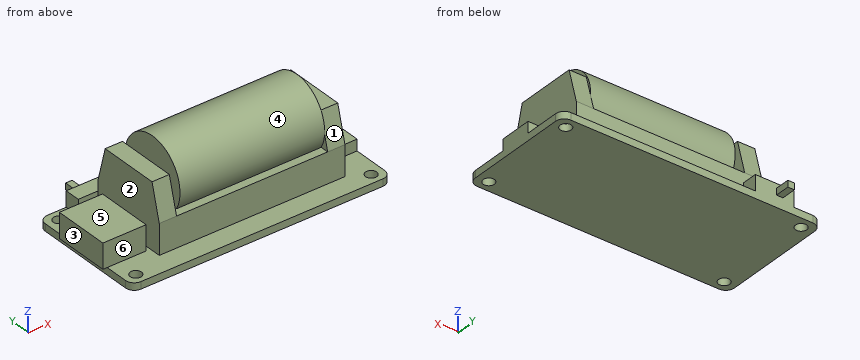
Autodesk Fusion 360 part; units mm, degrees
sketch "Sketch1" plane through (0, 0, 0) normal (0, 0, 1) x (1, 0, 0)
  line L0 (2, 0) -> (58, 0)
  line L1 (60, 2) -> (60, 26)
  line L2 (58, 28) -> (2, 28)
  line L3 (0, 26) -> (0, 2)
  arc A0 (2, 28) -> (0, 26) centre (2, 26) ccw
  arc A1 (60, 26) -> (58, 28) centre (58, 26) ccw
  arc A2 (58, 0) -> (60, 2) centre (58, 2) ccw
  arc A3 (0, 2) -> (2, 0) centre (2, 2) ccw
  point P0 (60, 0)
  point P1 (0, 28)
  dimension "d56" = 60
  dimension "d57" = 28
  dimension "d58" = 2
extrude "Extrude1" add sketch "Sketch1" along normal blind 1.65
sketch "Sketch2" plane through (0, 0, 1.65) normal (0, 0, 1) x (-1, 0, 0)
  arc A0 (0, -2) -> (-2, 0) centre (-2, -2) ccw
  line L0 (-2, 0) -> (-58, 0)
  arc A1 (-58, 0) -> (-60, -2) centre (-58, -2) ccw
  line L1 (-60, -2) -> (-60, -26)
  arc A2 (-60, -26) -> (-58, -28) centre (-58, -26) ccw
  line L2 (-58, -28) -> (-2, -28)
  arc A3 (-2, -28) -> (0, -26) centre (-2, -26) ccw
  line L3 (0, -26) -> (0, -2)
  line L4 (1, -20.5) -> (-9, -20.5)
  line L5 (-9, -20.5) -> (-9, -7.5)
  line L6 (-9, -7.5) -> (1, -7.5)
  line L7 (1, -7.5) -> (1, -20.5)
  line L8 (0, -14) -> (-60, -14) construction
  dimension "d61" = 10
  dimension "d62" = 13
  dimension "d63" = 1
extrude "Extrude2" add sketch "Sketch2" along normal blind 5.75 contours L3 L4 L6 L7 | L3 L4 L5 L6
sketch "Sketch3" plane through (0, 0, 1.65) normal (0, 0, 1) x (-1, 0, 0)
  line L0 (-9, -7.5) -> (0, -7.5)
  line L1 (0, -7.5) -> (0, -2)
  arc A0 (0, -2) -> (-2, 0) centre (-2, -2) ccw
  line L2 (-2, 0) -> (-58, 0)
  arc A1 (-58, 0) -> (-60, -2) centre (-58, -2) ccw
  line L3 (-60, -2) -> (-60, -26)
  arc A2 (-60, -26) -> (-58, -28) centre (-58, -26) ccw
  line L4 (-58, -28) -> (-2, -28)
  arc A3 (-2, -28) -> (0, -26) centre (-2, -26) ccw
  line L5 (0, -26) -> (0, -20.5)
  line L6 (0, -20.5) -> (-9, -20.5)
  line L7 (-9, -20.5) -> (-9, -7.5)
  line L8 (-9, -14) -> (-60, -14) construction
  line L9 (-10, -23.15) -> (-53, -23.15)
  line L10 (-53, -23.15) -> (-53, -4.85)
  line L11 (-53, -4.85) -> (-10, -4.85)
  line L12 (-10, -4.85) -> (-10, -23.15)
  dimension "d66" = 43
  dimension "d67" = 18.3
  dimension "d68" = 1
extrude "Extrude3" add sketch "Sketch3" along normal blind 15 contours L9 L10 L11 L12
sketch "Sketch4" plane through (53, 0, 0) normal (1, 0, 0) x (0, 1, 0)
  line L0 (4.85, 1.65) -> (23.15, 1.65)
  line L1 (23.15, 1.65) -> (23.15, 16.65)
  line L2 (23.15, 16.65) -> (4.85, 16.65)
  line L3 (4.85, 16.65) -> (4.85, 1.65)
  line L4 (4.85, 8.65) -> (7.2688, 17.65)
  line L5 (7.2688, 17.65) -> (20.7313, 17.65)
  line L6 (20.7313, 17.65) -> (23.15, 8.65)
  line L7 (4.85, 8.65) -> (23.15, 8.65) construction
  line L8 (7, 16.65) -> (21, 16.65) construction
  line L9 (14, 16.65) -> (14, 1.65) construction
  dimension "d71" = 14
  dimension "d72" = 7
  dimension "d73" = 1
extrude "Extrude4" cut sketch "Sketch4" against normal up to surface (43 mm away) contours L2 L3 L4 | L1 L2 L6
sketch "Sketch5" plane through (0, 4.85, 0) normal (0, -1, 0) x (1, 0, 0)
  line L0 (53, 8.65) -> (10, 8.65)
  line L1 (10, 8.65) -> (10, 1.65)
  line L2 (10, 1.65) -> (53, 1.65)
  line L3 (53, 1.65) -> (53, 8.65)
  line L4 (14, 16.65) -> (49, 16.65)
  line L5 (49, 16.65) -> (49, 8.65)
  line L6 (49, 8.65) -> (14, 8.65)
  line L7 (14, 8.65) -> (14, 16.65)
  line L8 (10, 8.65) -> (10, 16.65)
  line L9 (31.5, 1.65) -> (31.5, 16.653) construction
  line L10 (10, 16.65) -> (53, 16.65) construction
  dimension "d76" = 4
extrude "Extrude5" cut sketch "Sketch5" against normal through all contours L0 L4 L5 L6 L7
sketch "Sketch6" plane through (0, 0, 8.65) normal (0, 0, 1) x (-1, 0, 0)
  line L0 (-49, -23.15) -> (-14, -23.15)
  line L1 (-14, -23.15) -> (-14, -4.85)
  line L2 (-14, -4.85) -> (-49, -4.85)
  line L3 (-49, -4.85) -> (-49, -23.15)
  line L4 (-14, -14) -> (-49, -14) construction
  line L5 (-14, -21.15) -> (-49, -21.15)
  line L6 (-49, -21.15) -> (-49, -6.85)
  line L7 (-49, -6.85) -> (-14, -6.85)
  line L8 (-14, -6.85) -> (-14, -21.15)
  dimension "d78" = 2
extrude "Extrude6" cut sketch "Sketch6" against normal blind 6 contours L1 L3 L5 L6 L7 L8
sketch "Sketch7" plane through (49, 0, 0) normal (-1, 0, 0) x (0, -1, 0)
  line L0 (-4.85, 8.65) -> (-7, 16.65)
  line L1 (-7, 16.65) -> (-21, 16.65)
  line L2 (-21, 16.65) -> (-23.15, 8.65)
  line L3 (-23.15, 8.65) -> (-21.15, 8.65)
  line L4 (-21.15, 8.65) -> (-21.15, 2.65)
  line L5 (-21.15, 2.65) -> (-6.85, 2.65)
  line L6 (-6.85, 2.65) -> (-6.85, 8.65)
  line L7 (-6.85, 8.65) -> (-4.85, 8.65)
  line L8 (-14, 16.65) -> (-14, 2.65) construction
  circle A0 centre (-14, 12.65) radius 8.25
  dimension "d81" = 16.5
  dimension "d82" = 4
extrude "Extrude7" add sketch "Sketch7" along normal blind 33.5 contours L0 L1 L2 L3 L4 L6 L7 A0 | L0 L1 L2 A0
sketch "Sketch8" plane through (0, 0, 1.65) normal (0, 0, 1) x (-1, 0, 0)
  line L0 (-10, -4.85) -> (-10, -23.15)
  line L1 (-10, -23.15) -> (-53, -23.15)
  line L2 (-53, -23.15) -> (-53, -4.85)
  line L3 (-53, -4.85) -> (-10, -4.85)
  line L4 (-9, -7.5) -> (0, -7.5)
  line L5 (0, -7.5) -> (0, -2)
  arc A0 (0, -2) -> (-2, 0) centre (-2, -2) ccw
  line L6 (-2, 0) -> (-58, 0)
  arc A1 (-58, 0) -> (-60, -2) centre (-58, -2) ccw
  line L7 (-60, -2) -> (-60, -26)
  arc A2 (-60, -26) -> (-58, -28) centre (-58, -26) ccw
  line L8 (-58, -28) -> (-2, -28)
  arc A3 (-2, -28) -> (0, -26) centre (-2, -26) ccw
  line L9 (0, -26) -> (0, -20.5)
  line L10 (0, -20.5) -> (-9, -20.5)
  line L11 (-9, -20.5) -> (-9, -7.5)
  line L12 (-60, -14) -> (-9, -14) construction
  line L13 (-60, -17.75) -> (-54.4, -17.75)
  line L14 (-54.4, -17.75) -> (-54.4, -10.25)
  line L15 (-54.4, -10.25) -> (-60, -10.25)
  line L16 (-60, -10.25) -> (-60, -17.75)
  dimension "d85" = 5.6
  dimension "d86" = 7.5
extrude "Extrude8" add sketch "Sketch8" along normal blind 2.6 contours L7 L13 L14 L15 L16
sketch "Sketch9" plane through (0, 0, 0) normal (0, 0, -1) x (1, 0, 0)
  arc A0 (2, 0) -> (0, -2) centre (2, -2) ccw
  line L0 (0, -2) -> (0, -26)
  arc A1 (0, -26) -> (2, -28) centre (2, -26) ccw
  line L1 (2, -28) -> (58, -28)
  arc A2 (58, -28) -> (60, -26) centre (58, -26) ccw
  line L2 (60, -26) -> (60, -2)
  arc A3 (60, -2) -> (58, 0) centre (58, -2) ccw
  line L3 (58, 0) -> (2, 0)
  line L4 (0, -14) -> (60, -14) construction
  line L5 (30, 0) -> (30, -28) construction
  circle A4 centre (2.75, -2.5) radius 1.3
  circle A5 centre (57.25, -2.5) radius 1.3
  circle A6 centre (2.75, -25.5) radius 1.3
  circle A7 centre (57.25, -25.5) radius 1.3
  line L6 (2.75, -2.5) -> (57.25, -2.5) construction
  line L7 (57.25, -2.5) -> (57.25, -25.5) construction
  line L8 (57.25, -25.5) -> (2.75, -25.5) construction
  line L9 (2.75, -25.5) -> (2.75, -2.5) construction
  dimension "d89" = 23
  dimension "d90" = 54.5
  dimension "d91" = 2.6
extrude "Extrude9" cut sketch "Sketch9" against normal up to surface (1.65 mm away) contours A4 | A5 | A6 | A7
sketch "Sketch10" plane through (0, 0, 1.65) normal (0, 0, 1) x (-1, 0, 0)
  circle A0 centre (-57.25, -2.5) radius 1.3
  circle A1 centre (-57.25, -25.5) radius 1.3
  circle A2 centre (-2.75, -2.5) radius 1.3
  circle A3 centre (-2.75, -25.5) radius 1.3
  line L0 (-54.4, -17.75) -> (-60, -17.75)
  line L1 (-60, -17.75) -> (-60, -26)
  arc A4 (-60, -26) -> (-58, -28) centre (-58, -26) ccw
  line L2 (-58, -28) -> (-2, -28)
  arc A5 (-2, -28) -> (0, -26) centre (-2, -26) ccw
  line L3 (0, -26) -> (0, -20.5)
  line L4 (0, -20.5) -> (-9, -20.5)
  line L5 (-9, -20.5) -> (-9, -7.5)
  line L6 (-9, -7.5) -> (0, -7.5)
  line L7 (0, -7.5) -> (0, -2)
  arc A6 (0, -2) -> (-2, 0) centre (-2, -2) ccw
  line L8 (-2, 0) -> (-58, 0)
  arc A7 (-58, 0) -> (-60, -2) centre (-58, -2) ccw
  line L9 (-60, -2) -> (-60, -10.25)
  line L10 (-60, -10.25) -> (-54.4, -10.25)
  line L11 (-54.4, -10.25) -> (-54.4, -17.75)
  line L12 (-10, -4.85) -> (-10, -23.15)
  line L13 (-10, -23.15) -> (-53, -23.15)
  line L14 (-53, -23.15) -> (-53, -4.85)
  line L15 (-53, -4.85) -> (-10, -4.85)
  line L16 (-6.4, -28) -> (-15.3, -28)
  line L17 (-15.3, -28) -> (-15.3, -24.4)
  line L18 (-15.3, -24.4) -> (-6.4, -24.4)
  line L19 (-6.4, -24.4) -> (-6.4, -28)
  dimension "d1" = 8.9
  dimension "d2" = 3.6
  dimension "d3" = 15.3
extrude "Extrude10" add sketch "Sketch10" along normal blind 3.6 contours L2 L16 L17 L18 L19
sketch "Sketch11" plane through (0, 28, 0) normal (0, 1, 0) x (-1, 0, 0)
  line L0 (-58, 0) -> (-2, 0)
  line L1 (-2, 0) -> (-2, 1.65)
  line L2 (-2, 1.65) -> (-6.4, 1.65)
  line L3 (-6.4, 1.65) -> (-6.4, 5.25)
  line L4 (-6.4, 5.25) -> (-15.3, 5.25)
  line L5 (-15.3, 5.25) -> (-15.3, 1.65)
  line L6 (-15.3, 1.65) -> (-58, 1.65)
  line L7 (-58, 1.65) -> (-58, 0)
  line L8 (-15.3, 3.45) -> (-6.4, 3.45) construction
  line L9 (-8.9, 2.7) -> (-10.4, 2.7)
  line L10 (-10.4, 2.7) -> (-10.4, 4.2)
  line L11 (-10.4, 4.2) -> (-8.9, 4.2)
  line L12 (-8.9, 4.2) -> (-8.9, 2.7)
  line L13 (-8.9, 2.7) -> (-10.4, 4.2) construction
  line L14 (-10.4, 2.7) -> (-8.9, 4.2) construction
  point P0 (-9.65, 3.45)
  dimension "d6" = 1.5
  dimension "d7" = 1.5
  dimension "d8" = 2.5
extrude "Extrude11" add sketch "Sketch11" along normal blind 3.4 contours L9 L10 L11 L12
Check sheet for the modelled part. Datum: model origin and axes. Units: mm. Face numbers are marked on the shaded views. A direction names the side the tool comes from. Round coordinates to 2 decimals unless told otherwise and drop trailing zeros. Order: outer loops, then holes, each group sorted by start corner. A loop starts at its lowest first (then second) coordinate and runs counter-clockwise, first axis right, second up.
1) Section check C-C (x = 2.75). Record the boundary of the cut face in (y, z), and give its area (3 significant figures).
2) Scan lines: line 1 (X direction, y = 16, z = 4.5); line 2 (Y direction, x = 57.25, z = 0.9); line 3 (X direction, y = 9.5, z = 13.5). Record each from-to range of solid material in increasing order.
3) Go/stop test with flat-tipped pins: pin 1 Ø6.5 at (x, z) = (3.5, 4) entering from +Y; pin 2 Ø2 at (y, z) = (9, 7.5) entering from +X; pin 3 Ø1.6 at (y, z) = (30.5, 3.5) entering from +X. Record where each tip stops, or that it passes through.
4) Section check D-D (y = 13.5). Record the boundary of the cut face in (x, z).
5) Section check B-B (z = 15.25). Record the boundary of the cut face in (x, y).
6) Section check A-A (x = 30). Record the boundary of the cut face in (y, z).
7) Tool access check on the marked faces 4, 5 and 6. Record the directions out of +Z, -Z, +X, -X, +Y, -Y that give a thin tool (end or side, any length) a straight path to the whole face; none if there is none.
8) Mould release check, pull along X, two halves, no side actions. Record for the marked faces 1, 2 and 3: +X half, -X half, draft (parallel to the pull), parting line (faces both ways), or undercut.
Result:
1. outline: (0, 0) - (1.2, 0) - (1.2, 1.65) - (0, 1.65) - close; (3.8, 0) - (24.2, 0) - (24.2, 1.65) - (20.5, 1.65) - (20.5, 7.4) - (7.5, 7.4) - (7.5, 1.65) - (3.8, 1.65) - close; (26.8, 0) - (28, 0) - (28, 1.65) - (26.8, 1.65) - close
1. area: 112 mm2
2. line 1: x = -1 to 9, 10 to 14, 49 to 53
2. line 2: y = 0 to 1.2, 3.8 to 24.2, 26.8 to 28
2. line 3: x = 10 to 14, 15.5 to 53
3. pin 1: stops at y = 28
3. pin 2: stops at x = 53
3. pin 3: stops at x = 10.4
4. outline: (-1, 1.65) - (0, 1.65) - (0, 0) - (60, 0) - (60, 4.25) - (54.4, 4.25) - (54.4, 1.65) - (53, 1.65) - (53, 16.65) - (49, 16.65) - (49, 20.88) - (15.5, 20.88) - (15.5, 4.42) - (49, 4.42) - (49, 2.65) - (14, 2.65) - (14, 16.65) - (10, 16.65) - (10, 1.65) - (9, 1.65) - (9, 7.4) - (-1, 7.4) - close
5. outline: (10, 6.62) - (14, 6.62) - (14, 21.38) - (10, 21.38) - close; (15.5, 6.17) - (49, 6.17) - (49, 6.62) - (53, 6.62) - (53, 21.38) - (49, 21.38) - (49, 21.83) - (15.5, 21.83) - close
6. outline: (0, 0) - (28, 0) - (28, 1.65) - (23.15, 1.65) - (23.15, 8.65) - (21.22, 8.65) arc R8.25 ccw (long way) to (6.78, 8.65) - (4.85, 8.65) - (4.85, 1.65) - (0, 1.65) - close; hole (6.85, 2.65) - (21.15, 2.65) - (21.15, 8.53) arc R8.25 cw to (6.85, 8.53) - close
7. face 4: none
7. face 5: +Z, -X, +Y, -Y
7. face 6: +Z, -X, -Y
8. face 1: draft
8. face 2: undercut
8. face 3: -X half
